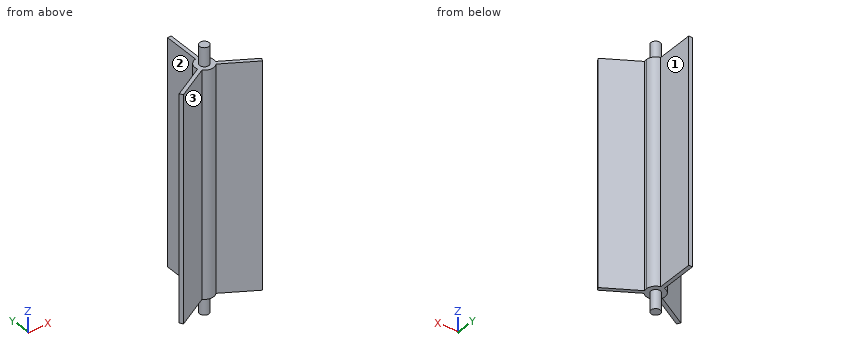
```python
from build123d import *

# Parameters (mm, degrees)
BOSS_EXTRUDE1_DEPTH      = 304.8
BOSS_EXTRUDE2_DEPTH      = 25.4
BOSS_EXTRUDE2_DEPTH_BACK = 330.2
SKETCH2_R                = 6.35


with BuildPart() as part:
    # Sketch1 → Boss-Extrude1 (new body)
    with BuildSketch(Plane.XY):
        with BuildLine():
            Line((-2.54, 1.466469684), (-2.54, 12.443407893))
            ThreePointArc((-2.54, 12.443407893), (-10.998522628, 6.35), (-12.046307345, -4.021999421))
            Line((-12.046307345, -4.021999421), (-2.54, 1.466469684))
        make_face()
        with BuildLine():
            ThreePointArc((-9.506307345, -8.421408472), (0, -12.7), (9.506307345, -8.421408472))
            Line((9.506307345, -8.421408472), (0, -2.932939367))
            Line((0, -2.932939367), (-9.506307345, -8.421408472))
        make_face()
        with BuildLine():
            ThreePointArc((12.7, 0), (9.837377699, 8.032185257), (2.54, 12.443407893))
            Line((2.54, 12.443407893), (2.54, 1.466469684))
            Line((2.54, 1.466469684), (12.046307345, -4.021999421))
            ThreePointArc((12.046307345, -4.021999421), (12.535511623, -2.037387631), (12.7, 0))
        make_face()
        with BuildLine():
            Line((10.998522628, -6.35), (0, 0))
            Line((0, 0), (-10.998522628, -6.35))
            ThreePointArc((-10.998522628, -6.35), (-10.304595884, -7.423294665), (-9.506307345, -8.421408472))
            Line((-9.506307345, -8.421408472), (0, -2.932939367))
            Line((0, -2.932939367), (9.506307345, -8.421408472))
            ThreePointArc((9.506307345, -8.421408472), (10.304595884, -7.423294665), (10.998522628, -6.35))
        make_face()
        with BuildLine():
            Line((-10.998522628, -6.35), (0, 0))
            Line((0, 0), (0, 12.7))
            ThreePointArc((0, 12.7), (-1.276463817, 12.635689143), (-2.54, 12.443407893))
            Line((-2.54, 12.443407893), (-2.54, 1.466469684))
            Line((-2.54, 1.466469684), (-12.046307345, -4.021999421))
            ThreePointArc((-12.046307345, -4.021999421), (-11.581059701, -5.212394479), (-10.998522628, -6.35))
        make_face()
        with BuildLine():
            Line((0, 12.7), (0, 0))
            Line((0, 0), (10.998522628, -6.35))
            ThreePointArc((10.998522628, -6.35), (11.581059701, -5.212394479), (12.046307345, -4.021999421))
            Line((12.046307345, -4.021999421), (2.54, 1.466469684))
            Line((2.54, 1.466469684), (2.54, 12.443407893))
            ThreePointArc((2.54, 12.443407893), (1.276463817, 12.635689143), (0, 12.7))
        make_face()
        with BuildLine():
            Line((0, 63.5), (0, 12.7))
            ThreePointArc((0, 12.7), (1.276463817, 12.635689143), (2.54, 12.443407893))
            Line((2.54, 12.443407893), (2.54, 63.5))
            Line((2.54, 63.5), (0, 63.5))
        make_face()
        with BuildLine():
            ThreePointArc((-2.54, 12.443407893), (-1.276463817, 12.635689143), (0, 12.7))
            Line((0, 12.7), (0, 63.5))
            Line((0, 63.5), (-2.54, 63.5))
            Line((-2.54, 63.5), (-2.54, 12.443407893))
        make_face()
        with BuildLine():
            Line((-54.99261314, -31.75), (-10.998522628, -6.35))
            ThreePointArc((-10.998522628, -6.35), (-11.581059701, -5.212394479), (-12.046307345, -4.021999421))
            Line((-12.046307345, -4.021999421), (-56.26261314, -29.550295474))
            Line((-56.26261314, -29.550295474), (-54.99261314, -31.75))
        make_face()
        with BuildLine():
            ThreePointArc((-9.506307345, -8.421408472), (-10.304595884, -7.423294665), (-10.998522628, -6.35))
            Line((-10.998522628, -6.35), (-54.99261314, -31.75))
            Line((-54.99261314, -31.75), (-53.72261314, -33.949704526))
            Line((-53.72261314, -33.949704526), (-9.506307345, -8.421408472))
        make_face()
        with BuildLine():
            Line((54.99261314, -31.75), (10.998522628, -6.35))
            ThreePointArc((10.998522628, -6.35), (10.304595884, -7.423294665), (9.506307345, -8.421408472))
            Line((9.506307345, -8.421408472), (53.72261314, -33.949704526))
            Line((53.72261314, -33.949704526), (54.99261314, -31.75))
        make_face()
        with BuildLine():
            ThreePointArc((12.046307345, -4.021999421), (11.581059701, -5.212394479), (10.998522628, -6.35))
            Line((10.998522628, -6.35), (54.99261314, -31.75))
            Line((54.99261314, -31.75), (56.26261314, -29.550295474))
            Line((56.26261314, -29.550295474), (12.046307345, -4.021999421))
        make_face()
    extrude(amount=BOSS_EXTRUDE1_DEPTH)

    # Sketch2 → Boss-Extrude2 (add, two sides: drawn at the far end of the back side and taken through both)
    with BuildSketch(Plane.XY.offset(304.8).offset(-BOSS_EXTRUDE2_DEPTH_BACK)):
        Circle(SKETCH2_R)
    extrude(amount=BOSS_EXTRUDE2_DEPTH + BOSS_EXTRUDE2_DEPTH_BACK)


solid = part.part
```
Design review of the part built by this model. Coordinates are the model's own, in mm. Face numbers are marked on the shaded views. Give positions to 0.01 mm unless a question says otherwise; leave off trailing zeros. Loops run counter-clockwise (first coordinate to the right, second up) from the corner with the lowest first, then second, coordinate; pieces in that order, holes last. Notation, with made-up numbers: M 4,6 L 31,6 A10 ccw 31,25 Z; hole C 13,-19.75 d2. An arc over 180 degrees is marked long. Return JSON: item names as keys, results as strings. Group by question number.
Item 1: Mouldability with a two-part tool opening along X and no side actions: class the marked faces 1, 2 and 3 as released by +X, released by -X, zero draft, split by the parting line, or undercut.
Item 2: Insertion check: pin 1 Ø1.5 at (x, z) = (-5, 208) entering from +Y; pin 2 Ø2 at (y, z) = (17.5, 43) entering from +X; pin 3 Ø1 at (y, z) = (9.5, 176.5) entering from +X. Each pin has a flat end and moves straight along its axis. Give the tip position at first contact, or say it passes through.
Item 3: We need section A-A (z = 205.5). Give the boundary of the cut face in (x, y).
Item 4: We need section C-C (z = 308.5). Give the boundary of the cut face in (x, y).
Item 5: For probe 1 along X at (y, z) = (13, 281); probe 2 along X at (y, z) = (4, 189); probe 3 along Z at (x, y) = (5, 11.5), list the stretches that pass through material, from the lowest coordinate up.
Item 6: We need section B-B (y = 23). Give the boundary of the cut face in (x, z).
Output:
{
 "1": {"face 1": "released by +X", "face 2": "released by -X", "face 3": "undercut"},
 "2": {"pin 1": "stops at y = 11.97", "pin 2": "stops at x = 2.54", "pin 3": "stops at x = 8.96"},
 "3": {"outline": "M -56.26,-29.55 L -53.72,-33.95 L -9.51,-8.42 A12.7 ccw 9.51,-8.42 L 53.72,-33.95 L 56.26,-29.55 L 12.05,-4.02 A12.7 ccw 2.54,12.44 L 2.54,63.5 L -2.54,63.5 L -2.54,12.44 A12.7 ccw -12.05,-4.02 Z"},
 "4": {"outline": "C 0,0 d12.7"},
 "5": {"probe 1": "x = -2.54 to 2.54", "probe 2": "x = -12.05 to 12.05", "probe 3": "z = 0 to 304.8"},
 "6": {"outline": "M -2.54,0 L 2.54,0 L 2.54,304.8 L -2.54,304.8 Z"}
}
